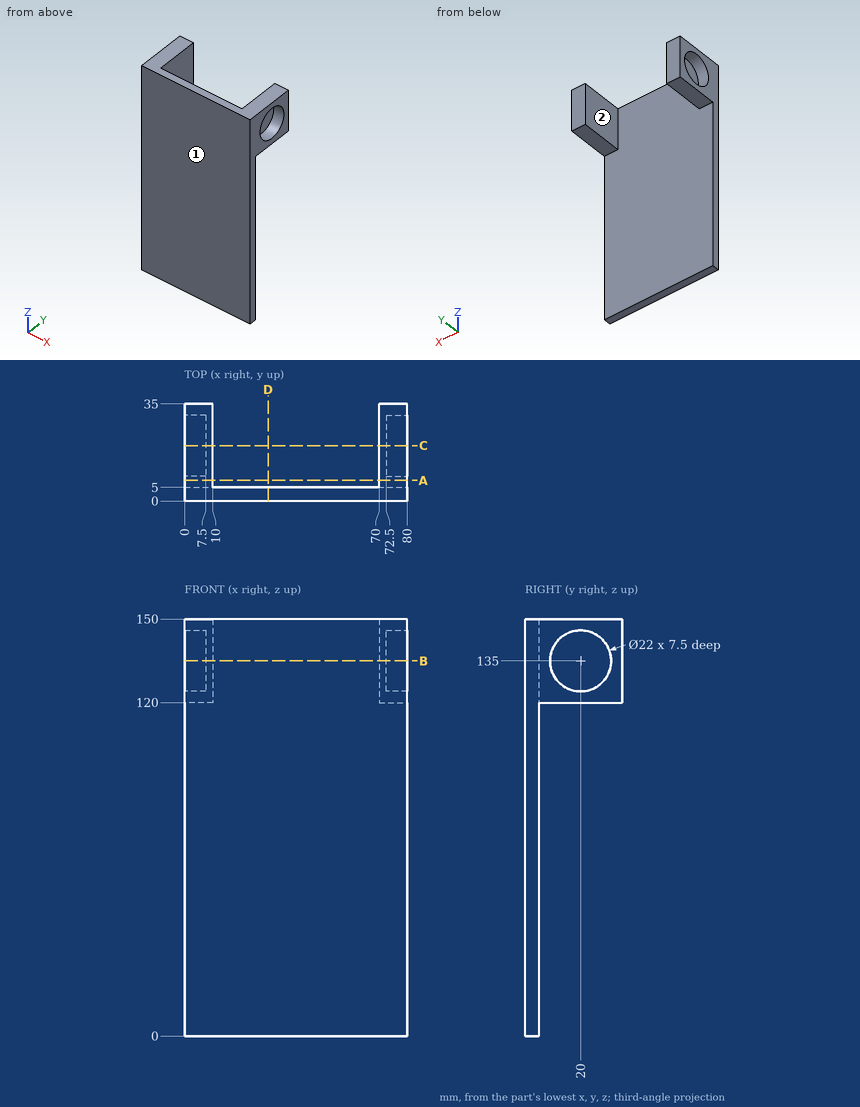
Design review of the part shown in the three views and the two pictorial views. Dimensions are in mm from the part's minimum x, y and z. Coordinates: 2 decimals unless noted, no trailing zeros. Order: outer loops, then holes, each group sorted by start corner. A loop starts at its lowest first (then second) coordinate and runs counter-clockwise, first axis right, second up.
1) Mouldability with a two-part tool opening along X and no side actions: class the marked faces 1 and 2 as +X half, -X half, draft (parallel to the pull), parting line (faces both ways), or undercut.
2) Take a section at B-B, the plane z = 135. Give the boundary of the cut face in (x, y).
3) Take a section at D-D, the plane x = 30. Give the boundary of the cut face in (y, z).
4) Take a section at A-A, the plane y = 7.5. Give the boundary of the cut face in (x, z).
5) Take a section at C-C, the plane y = 20. Give the boundary of the cut face in (x, z), and give its area (3 significant figures).
6) Wall thickness on line 1 along Y through (x, z) = (75.75, 135); line 2 along X through (y, z) = (9, 143); line 3 along Z through (x, y) = (5, 19.5): over which ranges is each line inside the solid? List them lowest first.
7) Clearance check with flat-ended pins moving along their axes: pin 1 (13 mm diameter, centred on y = 20, z = 135, fed in from +X); pin 2 (4 mm diameter, centred on x = 63, z = 119, fed in from +Y); pin 3 (11 mm diameter, centred on x = 7, y = 14.5, fed in from -Z). State where each tip first meets the part, or that it passes through.
Returned:
1. face 1: draft
1. face 2: undercut
2. outline: (0, 0) - (80, 0) - (80, 9) - (72.5, 9) - (72.5, 31) - (80, 31) - (80, 35) - (70, 35) - (70, 5) - (10, 5) - (10, 35) - (0, 35) - (0, 31) - (7.5, 31) - (7.5, 9) - (0, 9) - close
3. outline: (0, 0) - (5, 0) - (5, 150) - (0, 150) - close
4. outline: (0, 120) - (10, 120) - (10, 150) - (0, 150) - close; (70, 120) - (80, 120) - (80, 150) - (70, 150) - close
5. outline: (0, 120) - (10, 120) - (10, 150) - (0, 150) - (0, 146) - (7.5, 146) - (7.5, 124) - (0, 124) - close; (70, 120) - (80, 120) - (80, 124) - (72.5, 124) - (72.5, 146) - (80, 146) - (80, 150) - (70, 150) - close
5. area: 270 mm2
6. line 1: y = 0 to 9, 31 to 35
6. line 2: x = 0 to 10, 70 to 80
6. line 3: z = 120 to 124.01, 145.99 to 150
7. pin 1: stops at x = 72.5
7. pin 2: stops at y = 5
7. pin 3: stops at z = 120
